Read the model definition and answer for the solid it produces. Units are mm, in the model's axes. Face numbers are marked on the shaded views. A direction names the side the tool comes from. Round coordinates to 2 decimals unless told otherwise and drop trailing zeros. Write each loop counter-clockwise with the first axis right and the second up, starting at its lowest first coordinate (ties: lowest second). Pieces come first, ordered by that corner, then holes. Notation, with made-up numbers: (-27.75, 40.5) - (11.25, 40.5) arc R7 cw to (11.25, 53.5) - close; hole circle Ø4 at (-33, 9.25). An arc over 180 degrees is marked (long way). One line per item, written item: value. Start each with the question number.
(1) Flat-ended cylindrical pins translate along their axes: pin 1 Ø2.5 at (x, z) = (2, 2.5) entering from -Y (3 decimals); pin 2 Ø2 at (x, z) = (-11, 4.5) entering from +Y; pin 3 Ø2 at (y, z) = (-2.5, 5) entering from -X; pin 4 Ø2.5 at (x, z) = (-2, 2.5) entering from +Y (3 decimals). Find the tip coordinate at first contact, or state that the pin passes through.
(2) Find the intervals of material crossed by L1, parallel to X at y = 3.5, z = 1.5; L2, parallel to Y at x = -12.5, z = 0.3; L3, parallel to Y at x = 6, z = 1.5 (3 decimals), in increasing order.
(3) A cutting plane is placed at B-B, the plane z = 3.5. Determine the outline of the cut face in (x, y) (3 decimals).
(4) A cutting plane is placed at C-C, the plane x = -12.5. Determine the outline of the cut face in (y, z).
(5) For the marked faces 1, 2, 3 and 4, determine the directions among +Z, -Z, +X, -X, +Y, -Y from which every point of the face is accessible in a straight line to the end or side of a thin tool.
(6) The mould has two halves that part along Y. Classify the marked faces 5, 6, 7 and 8: +Y half, -Y half, draft (parallel to the pull), parting line (faces both ways), or undercut.
(7) A cutting plane is placed at D-D, the plane y = 0. State how many separate pieces and enclosed holes the cut face has, plus the area to 3 significant figures.
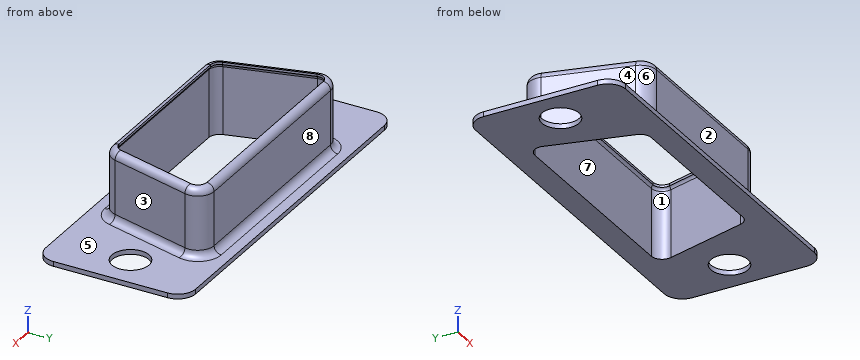
from build123d import *

# Parameters (mm, degrees)
SKETCH1_R           = 1.55
BOSS_EXTRUDE1_DEPTH = 0.4
BOSS_EXTRUDE2_DEPTH = 5.7
FILLET1_R           = 0.6
CUT_EXTRUDE1_DEPTH  = 5.9
FILLET2_R           = 0.3


# Some blends are built 0.0001 mm under size
with BuildPart() as part:
    # Sketch1 → Boss-Extrude1 (new body)
    with BuildSketch(Plane.XY):
        with BuildLine():
            Line((-13.95, 6.25), (13.95, 6.25))
            ThreePointArc((13.95, 6.25), (15.010660172, 5.810660172), (15.45, 4.75))
            Line((15.45, 4.75), (15.45, -4.75))
            ThreePointArc((15.45, -4.75), (15.010660172, -5.810660172), (13.95, -6.25))
            Line((13.95, -6.25), (-13.95, -6.25))
            ThreePointArc((-13.95, -6.25), (-15.010660172, -5.810660172), (-15.45, -4.75))
            Line((-15.45, -4.75), (-15.45, 4.75))
            ThreePointArc((-15.45, 4.75), (-15.010660172, 5.810660172), (-13.95, 6.25))
        make_face()
        with Locations((-12.5, 0)):
            Circle(SKETCH1_R, mode=Mode.SUBTRACT)
        with Locations((12.5, 0)):
            Circle(SKETCH1_R, mode=Mode.SUBTRACT)
        with BuildLine():
            Line((-8.611007598, 4.175), (8.611007598, 4.175))
            ThreePointArc((8.611007598, 4.175), (9.206022604, 3.881571072), (9.335451968, 3.230885716))
            Line((9.335451968, 3.230885716), (7.5, -3.619114284))
            ThreePointArc((7.5, -3.619114284), (7.232126702, -4.020015005), (6.77555563, -4.175))
            Line((6.77555563, -4.175), (-6.77555563, -4.175))
            ThreePointArc((-6.77555563, -4.175), (-7.232126702, -4.020015005), (-7.5, -3.619114284))
            Line((-7.5, -3.619114284), (-9.335451968, 3.230885716))
            ThreePointArc((-9.335451968, 3.230885716), (-9.206022604, 3.881571072), (-8.611007598, 4.175))
        make_face(mode=Mode.SUBTRACT)
    extrude(amount=BOSS_EXTRUDE1_DEPTH)

    # Sketch2 → Boss-Extrude2 (add)
    with BuildSketch(Plane.XY.offset(0.4)):
        with BuildLine():
            Line((-6.77555563, -4.775), (6.77555563, -4.775))
            ThreePointArc((6.77555563, -4.775), (7.597383559, -4.496027009), (8.079555496, -3.774405711))
            Line((8.079555496, -3.774405711), (9.915007464, 3.075594289))
            ThreePointArc((9.915007464, 3.075594289), (9.682034608, 4.246827929), (8.611007598, 4.775))
            Line((8.611007598, 4.775), (-8.611007598, 4.775))
            ThreePointArc((-8.611007598, 4.775), (-9.682034608, 4.246827929), (-9.915007464, 3.075594289))
            Line((-9.915007464, 3.075594289), (-8.079555496, -3.774405711))
            ThreePointArc((-8.079555496, -3.774405711), (-7.597383559, -4.496027009), (-6.77555563, -4.775))
        make_face()
        with BuildLine():
            Line((-6.77555563, -4.175), (6.77555563, -4.175))
            ThreePointArc((6.77555563, -4.175), (7.232126702, -4.020015005), (7.5, -3.619114284))
            Line((7.5, -3.619114284), (9.335451968, 3.230885716))
            ThreePointArc((9.335451968, 3.230885716), (9.206022604, 3.881571072), (8.611007598, 4.175))
            Line((8.611007598, 4.175), (-8.611007598, 4.175))
            ThreePointArc((-8.611007598, 4.175), (-9.206022604, 3.881571072), (-9.335451968, 3.230885716))
            Line((-9.335451968, 3.230885716), (-7.5, -3.619114284))
            ThreePointArc((-7.5, -3.619114284), (-7.232126702, -4.020015005), (-6.77555563, -4.175))
        make_face(mode=Mode.SUBTRACT)
    extrude(amount=BOSS_EXTRUDE2_DEPTH)

    # Fillet1
    fillet1_edges = [part.edges().sort_by_distance(p)[0] for p in [
        (-7.597383559, -4.496027009, 6.1),
        (0, -4.775, 6.1),
        (7.597383559, -4.496027009, 6.1),
        (8.99728148, -0.349405711, 6.1),
        (9.682034608, 4.246827929, 6.1),
        (0, 4.775, 6.1),
        (-9.682034608, 4.246827929, 6.1),
        (-8.99728148, -0.349405711, 6.1),
        (-7.597383559, -4.496027009, 0.4),
        (0, -4.775, 0.4),
        (7.597383559, -4.496027009, 0.4),
        (8.99728148, -0.349405711, 0.4),
        (9.682034608, 4.246827929, 0.4),
        (0, 4.775, 0.4),
        (-9.682034608, 4.246827929, 0.4),
        (-8.99728148, -0.349405711, 0.4),
    ]]
    fillet(fillet1_edges, radius=FILLET1_R - 0.0001)  # a hair under: the kernel refuses the full size

    # Sketch3 → Cut-Extrude1 (cut)
    with BuildSketch(Plane(origin=(0, 0, 0), x_dir=(-1, 0, 0), z_dir=(0, 0, -1))):
        with BuildLine():
            Line((-6.77555563, -4.325), (6.77555563, -4.325))
            ThreePointArc((6.77555563, -4.325), (7.323440916, -4.139018006), (7.644888874, -3.657937141))
            Line((7.644888874, -3.657937141), (9.480340842, 3.192062859))
            ThreePointArc((9.480340842, 3.192062859), (9.325025605, 3.972885286), (8.611007598, 4.325))
            Line((8.611007598, 4.325), (-8.611007598, 4.325))
            ThreePointArc((-8.611007598, 4.325), (-9.325025605, 3.972885286), (-9.480340842, 3.192062859))
            Line((-9.480340842, 3.192062859), (-7.644888874, -3.657937141))
            ThreePointArc((-7.644888874, -3.657937141), (-7.323440916, -4.139018006), (-6.77555563, -4.325))
        make_face()
    extrude(amount=-CUT_EXTRUDE1_DEPTH, mode=Mode.SUBTRACT)

    # Fillet2
    # the kernel refuses this fillet: 0.3 mm, written as the material it adds along each edge
    with BuildSketch(Plane(origin=(6.77555563, -3.425, 5.9), x_dir=(0.9659258262890676, -0.2588190451025228, 0), z_dir=(0.2588190451025228, 0.9659258262890676, 0))) as fillet2_piece_1:
        with BuildLine():
            CenterArc((0.6, 0.259807621), FILLET2_R, 300, 60)
            Line((0.75, 0), (0.753, -0.005196152))
            ThreePointArc((0.753, -0.005196152), (0.825, -0.006), (0.9, -0.006))
            Line((0.9, -0.006), (0.906, 0))
            Line((0.906, 0), (0.906, 0.259807621))
            Line((0.906, 0.259807621), (0.9, 0.259807621))
        make_face()
    revolve(axis=Axis((6.77555563, -3.425, 5.9), (0, 0, -1)), revolution_arc=75)
    with BuildSketch(Plane(origin=(9.480340842, 3.192062859, 5.9), x_dir=(0, 0, -1), z_dir=(-0.25881904510252507, -0.9659258262890672, 0)), Plane(origin=(-7.644888874, -3.657937141, 5.9), x_dir=(0, 0, -1), z_dir=(-0.25881904510252135, 0.9659258262890682, 0))) as fillet2_piece_2:
        with BuildLine():
            CenterArc((0.259807621, -0.3), FILLET2_R, 90, 60)
            Line((0, -0.15), (-0.005196152, -0.147))
            ThreePointArc((-0.005196152, -0.147), (-0.006, -0.075), (-0.006, 0))
            Line((-0.006, 0), (0, 0.006))
            Line((0, 0.006), (0.259807621, 0.006))
            Line((0.259807621, 0.006), (0.259807621, 0))
        make_face()
    extrude(amount=7.091641836)
    with BuildSketch(Plane(origin=(8.611007598, 3.425, 5.9), x_dir=(0, 1, 0), z_dir=(-1, 0, 0))) as fillet2_piece_3:
        with BuildLine():
            CenterArc((0.6, 0.259807621), FILLET2_R, 300, 60)
            Line((0.75, 0), (0.753, -0.005196152))
            ThreePointArc((0.753, -0.005196152), (0.825, -0.006), (0.9, -0.006))
            Line((0.9, -0.006), (0.906, 0))
            Line((0.906, 0), (0.906, 0.259807621))
            Line((0.906, 0.259807621), (0.9, 0.259807621))
        make_face()
    revolve(axis=Axis((8.611007598, 3.425, 5.9), (0, 0, -1)), revolution_arc=105)
    with BuildSketch(Plane(origin=(-8.611007598, 4.325, 5.9), x_dir=(0, 0, -1), z_dir=(1, 0, 0))) as fillet2_piece_4:
        with BuildLine():
            CenterArc((0.259807621, -0.3), FILLET2_R, 90, 60)
            Line((0, -0.15), (-0.005196152, -0.147))
            ThreePointArc((-0.005196152, -0.147), (-0.006, -0.075), (-0.006, 0))
            Line((-0.006, 0), (0, 0.006))
            Line((0, 0.006), (0.259807621, 0.006))
            Line((0.259807621, 0.006), (0.259807621, 0))
        make_face()
    extrude(amount=17.222015197)
    with BuildSketch(Plane(origin=(-8.611007598, 3.425, 5.9), x_dir=(-0.9659258262890688, -0.25881904510251935, 0), z_dir=(0.25881904510251935, -0.9659258262890688, 0))) as fillet2_piece_5:
        with BuildLine():
            CenterArc((0.6, 0.259807621), FILLET2_R, 300, 60)
            Line((0.75, 0), (0.753, -0.005196152))
            ThreePointArc((0.753, -0.005196152), (0.825, -0.006), (0.9, -0.006))
            Line((0.9, -0.006), (0.906, 0))
            Line((0.906, 0), (0.906, 0.259807621))
            Line((0.906, 0.259807621), (0.9, 0.259807621))
        make_face()
    revolve(axis=Axis((-8.611007598, 3.425, 5.9), (0, 0, -1)), revolution_arc=105)
    with BuildSketch(Plane(origin=(-6.77555563, -3.425, 5.9), x_dir=(0, -1, 0), z_dir=(1, 0, 0))) as fillet2_piece_6:
        with BuildLine():
            CenterArc((0.6, 0.259807621), FILLET2_R, 300, 60)
            Line((0.75, 0), (0.753, -0.005196152))
            ThreePointArc((0.753, -0.005196152), (0.825, -0.006), (0.9, -0.006))
            Line((0.9, -0.006), (0.906, 0))
            Line((0.906, 0), (0.906, 0.259807621))
            Line((0.906, 0.259807621), (0.9, 0.259807621))
        make_face()
    revolve(axis=Axis((-6.77555563, -3.425, 5.9), (0, 0, -1)), revolution_arc=75)
    with BuildSketch(Plane(origin=(6.77555563, -4.325, 5.9), x_dir=(0, 0, -1), z_dir=(-1, 0, 0))) as fillet2_piece_7:
        with BuildLine():
            CenterArc((0.259807621, -0.3), FILLET2_R, 90, 60)
            Line((0, -0.15), (-0.005196152, -0.147))
            ThreePointArc((-0.005196152, -0.147), (-0.006, -0.075), (-0.006, 0))
            Line((-0.006, 0), (0, 0.006))
            Line((0, 0.006), (0.259807621, 0.006))
            Line((0.259807621, 0.006), (0.259807621, 0))
        make_face()
    extrude(amount=13.551111261)


solid = part.part
Here are the results:
1. pin 1: y = -4.775
1. pin 2: through
1. pin 3: x = -8.69
1. pin 4: y = 4.775
2. L1: -9.96 to -9.51, 9.51 to 9.96
2. L2: -6.25 to -1.55, 1.55 to 6.25
2. L3: -4.775 to -4.325, 4.325 to 4.775
3. outline: (-9.915, 3.076) - (-8.08, -3.774) arc R1.35 ccw to (-6.776, -4.775) - (6.776, -4.775) arc R1.35 ccw to (8.08, -3.774) - (9.915, 3.076) arc R1.35 ccw to (8.611, 4.775) - (-8.611, 4.775) arc R1.35 ccw to start; hole (-9.48, 3.192) - (-7.645, -3.658) arc R0.9 ccw to (-6.776, -4.325) - (6.776, -4.325) arc R0.9 ccw to (7.645, -3.658) - (9.48, 3.192) arc R0.9 ccw to (8.611, 4.325) - (-8.611, 4.325) arc R0.9 ccw to start
4. outline: (-6.25, 0) - (-1.55, 0) - (-1.55, 0.4) - (-6.25, 0.4) - close; (1.55, 0) - (6.25, 0) - (6.25, 0.4) - (1.55, 0.4) - close
5. face 1: -Z
5. face 2: +Z, +X, -X, -Y
5. face 3: +Z, +X, -Y
5. face 4: +Z, -X, -Y
6. face 5: draft
6. face 6: -Y half
6. face 7: undercut
6. face 8: +Y half
7. separate pieces: 4
7. enclosed holes: 0
7. area: 8.38 mm²
